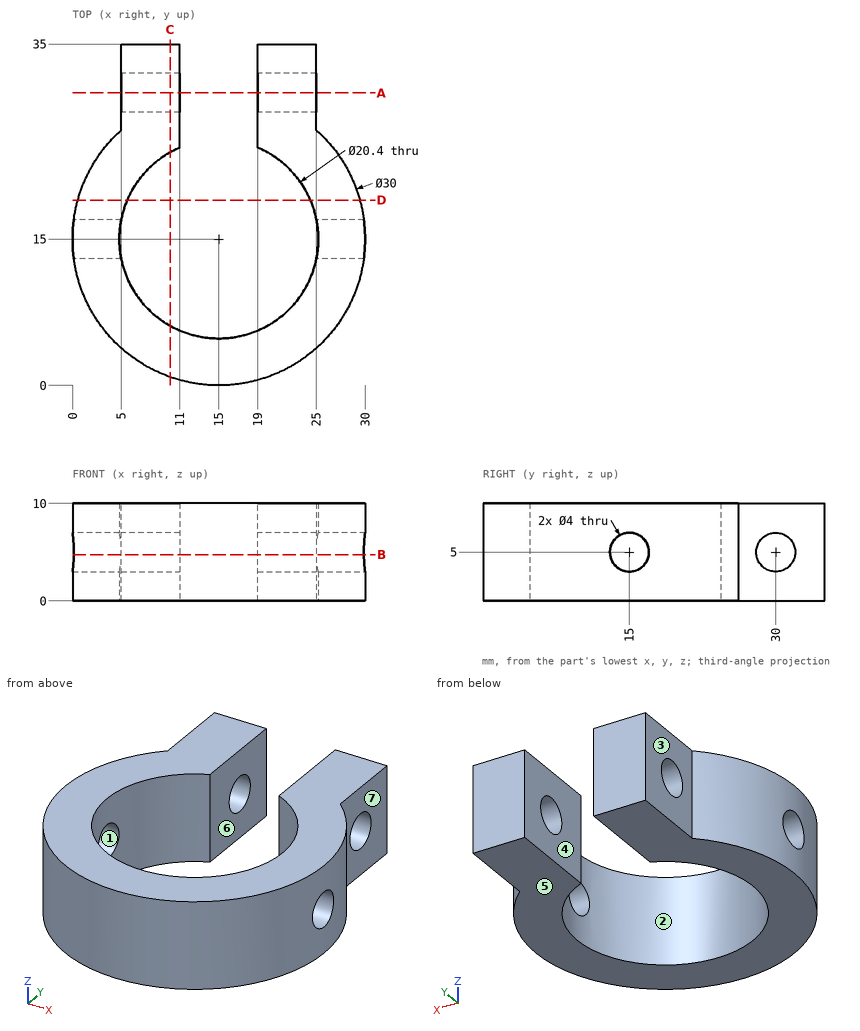
Can you work these out from the drawing? Everything is in mm from the part's minimum corner. A direction names the side the tool comes from. Coordinates: 2 decimals unless noted, no trailing zeros. Order: outer loops, then holes, each group sorted by start corner. A loop starts at its lowest first (then second) coordinate and runs counter-clockwise, first axis right, second up. Notation, with made-up numbers: M -26,-32.5 L -12,-32.5 A4 ccw -12,-25.5 Z; hole C -6.75,40.5 d3. An arc over 180 degrees is marked long. Answer as CSV lines item,"result". Start each with the question number.
1. We'd pull the mould along X, two halves only. Please class the marked faces 1, 2, 3 and 4: released by +X, released by -X, zero draft, split by the parting line, or undercut.
2. I want a section at B-B, the plane z = 4.75. Write out the boundary of the cut face in (x, y), and give its area (3 significant figures).
3. For pin 1 (6 mm diameter, centred on x = 10.5, z = 2.5, fed in from -Y); pin 2 (10 mm diameter, centred on x = 9.5, y = 19.5, fed in from -Z); pin 3 (2 mm diameter, centred on y = 30.5, z = 3.5, fed in from -X), each with a flat end and sliding along its axis, tell me the tip position at first contact or that it passes through.
4. On a 3-axis mill with a long thin cutter (end or side, diameter ignored), from which of +Z, -Z, +X, -X, +Y, -Y can I reach the whole of each face in a straight line? I mean the marked faces 5, 6 and 7. Say none if no direction works.
5. I need wall thicknesses on line 1 (X direction, y = 28, z = 6.75); line 2 (Y direction, x = 22.95, z = 5); line 3 (X direction, y = 26, z = 2.5). Which ranges of each line are inside material? Lowest first, please. Write a range as [from, to].
6. I want a section at A-A, the plane y = 30. Write out the boundary of the cut face in (x, z).
7. I want a section at D-D, the plane y = 19. Write out the boundary of the cut face in (x, z).
8. I want a section at C-C, the plane x = 10. Write out the boundary of the cut face in (y, z), and give its area (3 significant figures).
Recorded:
1,face 1,"zero draft"
1,face 2,"undercut"
1,face 3,"released by -X"
1,face 4,"undercut"
2,outline,"M 0.13,13.02 A15 ccw 29.87,13.02 L 25.01,13.02 A10.2 cw 4.99,13.02 Z; M 0.13,16.98 L 4.99,16.98 A10.2 cw 11,24.38 L 11,28.02 L 5,28.02 L 5,26.18 A15 ccw Z; M 5,31.98 L 11,31.98 L 11,35 L 5,35 Z; M 19,24.38 A10.2 cw 25.01,16.98 L 29.87,16.98 A15 ccw 25,26.18 L 25,28.02 L 19,28.02 Z; M 19,31.98 L 25,31.98 L 25,35 L 19,35 Z"
2,area,"338 mm2"
3,pin 1,"stops at y = 0.08"
3,pin 2,"stops at z = 0"
3,pin 3,"stops at x = 5"
4,face 5,"-Z, +X, -X, +Y, -Y"
4,face 6,"+Z, -Z, +Y"
4,face 7,"+Z, -Z, +X, +Y"
5,line 1,"x = [5, 11], [19, 25]"
5,line 2,"y = [2.28, 8.61], [21.39, 28], [32, 35]"
5,line 3,"x = [4.8, 11], [19, 25.2]"
6,outline,"M 5,0 L 11,0 L 11,3 L 5,3 Z; M 5,7 L 11,7 L 11,10 L 5,10 Z; M 19,0 L 25,0 L 25,3 L 19,3 Z; M 19,7 L 25,7 L 25,10 L 19,10 Z"
7,outline,"M 0.54,0 L 5.62,0 L 5.62,10 L 0.54,10 Z; M 24.38,0 L 29.46,0 L 29.46,10 L 24.38,10 Z"
8,outline,"M 0.86,0 L 6.11,0 L 6.11,10 L 0.86,10 Z; M 23.89,0 L 35,0 L 35,10 L 23.89,10 Z; hole C 30,5 d4"
8,area,"151 mm2"
